Verification items for the finished model (mm, model axes). A direction names the side the tool comes from. Round coordinates to 2 decimals unless told otherwise and drop trailing zeros. Order: outer loops, then holes, each group sorted by start corner. A loop starts at its lowest first (then second) coordinate and runs counter-clockwise, first axis right, second up. Notation, with made-up numbers: M 65,-18 L 71,-18 A17 ccw 71,8 Z; hole C -6,83 d3. An arc over 180 degrees is marked long. Return JSON: item names as keys, results as strings. Group by question number.
from build123d import *

# Parameters (mm, degrees)
EXTRUDE_1_DEPTH     = 18
SKETCH_3_R          = 4.15
SKETCH_3_W          = 2.5
SKETCH_3_H          = 12
EXTRUDE_2_DEPTH     = 4
SKETCH_4_R          = 5
CUT_EXTRUDE_1_DEPTH = 1


with BuildPart() as part:
    # 草图1 → 凸台-拉伸1 (new body)
    with BuildSketch(Plane.XY):
        with BuildLine():
            Line((13.754950724, 8.173208097), (11.36655926, 8.173208097))
            ThreePointArc((11.36655926, 8.173208097), (14, 0), (11.36655926, -8.173208097))
            Line((11.36655926, -8.173208097), (13.754950724, -8.173208097))
            ThreePointArc((13.754950724, -8.173208097), (16, 0), (13.754950724, 8.173208097))
        make_face()
    extrude(amount=EXTRUDE_1_DEPTH)

    # 草图3 → 凸台-拉伸2 (add)
    with BuildSketch(Plane(origin=(0, 0, 0), x_dir=(1, 0, 0), z_dir=(0, 1, 0))):
        with BuildLine():
            Line((17.25, -18), (14.877475362, -18))
            Line((14.877475362, -18), (14.877475362, 0))
            Line((14.877475362, 0), (17.25, 0))
            Line((17.25, 0), (28.186274783, -4.279138082))
            ThreePointArc((28.186274783, -4.279138082), (31.98307184, -10.317032459), (27.325150791, -15.718477442))
            Line((27.325150791, -15.718477442), (17.25, -18))
        make_face()
        with Locations(Location((26, -9.866642228, 0), (0, 0, 270))):
            Circle(SKETCH_3_R, mode=Mode.SUBTRACT)
        with Locations((17.25, -10.028578804)):
            Rectangle(SKETCH_3_W, SKETCH_3_H, mode=Mode.SUBTRACT)
    extrude(amount=EXTRUDE_2_DEPTH)

    # 草图4 → 切除-拉伸1 (cut)
    with BuildSketch(Plane(origin=(0, 4, 0), x_dir=(1, 0, 0), z_dir=(0, 1, 0))):
        with Locations(Location((26, -9.866642228, 0), (0, 0, 270))):
            Circle(SKETCH_4_R)
    extrude(amount=-CUT_EXTRUDE_1_DEPTH, mode=Mode.SUBTRACT)


solid = part.part
1. Cross-section at D-D (y = -1.5). Enter the section's corners in (x, z), plus the area to 3 significant figures.
2. Cross-section at B-B (z = 9.25). Enter the section's corners in (x, y), plus the area to 3 significant figures.
3. Draft check along X on faces 1 (the face through (14, 0, 9)), 2 (the face through (21, 0, 9)), 3 (the face through (18.5, 2, 10)). Enter one of: +X half, -X half, draft (parallel to the pull), parting line (faces both ways), or undercut.
4. Go/stop test with flat-tipped pins: pin 1 (5 mm diameter, centred on x = 21, z = 9.5, fed in from -Y); pin 2 (3 mm diameter, centred on y = 0.5, z = 15.5, fed in from +X); pin 3 (1.5 mm diameter, centred on y = -3.5, z = 8.5, fed in from +X). Record where each tip stops, or that it passes through.
5. Cross-section at C-C (x = 26). Enter the section's corners in (y, z), plus the area to 3 significant figures.
6. Cross-section at A-A (x = 16.75). Enter the section's corners in (y, z).
7. Access from +Z, -Z, +X, -X, +Y, -Y to the whole of each face (thin tool, end or side, straight path). Record for faces 4 (the face through (16, 2, 10)), 5 (the face through (14.3, -0.1, 18)), 6 (the face through (20.7, 4, 9.6)), 7 (the face through (30, 3, 8)), 8 (the face through (13, -8.173, 9)).
8. Thickness scan on line 1 along X through (y, z) = (3.5, 7); line 2 along X through (y, z) = (0.5, 10.5); line 3 along Z through (x, y) = (29.75, 1.5). Record the ranges inside material, lowest first. Write a range as from..to.
Computed:
{
 "1": {"outline": "M 13.92,0 L 15.93,0 L 15.93,18 L 13.92,18 Z", "area": "36.2 mm²"},
 "2": {"outline": "M 11.37,-8.17 L 13.75,-8.17 A16 ccw 16,0 L 16,4 L 15.49,4 A16 ccw 13.75,8.17 L 11.37,8.17 A14 cw Z; M 18.5,0 L 21.9,0 L 21.9,3 L 21.04,3 L 21.04,4 L 18.5,4 Z; M 30.1,0 L 31.97,0 L 31.97,4 L 30.96,4 L 30.96,3 L 30.1,3 Z", "area": "54.6 mm²"},
 "3": {"face 1": "-X half", "face 2": "draft", "face 3": "undercut"},
 "4": {"pin 1": "stops at y = 0", "pin 2": "stops at x = 30.35", "pin 3": "stops at x = 15.76"},
 "5": {"outline": "M 0,3.42 L 4,3.42 L 4,4.87 L 3,4.87 L 3,5.72 L 0,5.72 Z; M 0,14.02 L 3,14.02 L 3,14.87 L 4,14.87 L 4,16.02 L 0,16.02 Z", "area": "15.5 mm²"},
 "6": {"outline": "M 0,0 L 4,0 L 4,4.03 L 0,4.03 Z; M 0,16.03 L 4,16.03 L 4,18 L 0,18 Z"},
 "7": {"face 4": "+Y, -Y", "face 5": "+Z, +X, -X, +Y, -Y", "face 6": "+Z, -Z, +X, +Y", "face 7": "+Y", "face 8": "+Z, -Z, +X, -X, -Y"},
 "8": {"line 1": "x = 13.56..16, 18.5..21.9, 30.1..31.27", "line 2": "x = 13.99..16, 18.5..21.9, 30.1..31.97", "line 3": "z = 5.18..8.09, 11.64..14.55"}
}
